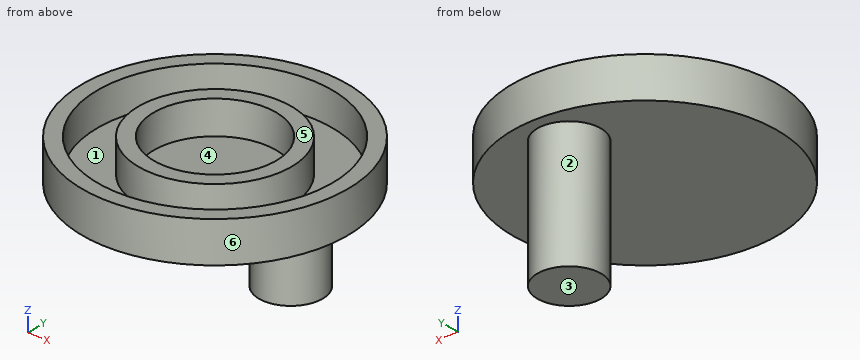
```python
from build123d import *

# Parameters (mm, degrees)
SKETCH1_R           = 12.5
BOSS_EXTRUDE1_DEPTH = 50
SKETCH2_R           = 52.025
SKETCH2_R_2         = 46.025
SKETCH2_R_3         = 29.975
SKETCH2_R_4         = 23.975
BOSS_EXTRUDE2_DEPTH = 16
SKETCH4_R           = 52.025
BOSS_EXTRUDE3_DEPTH = 3


with BuildPart() as part:
    # Sketch1 → Boss-Extrude1 (new body)
    with BuildSketch(Plane.XY):
        Circle(SKETCH1_R)
    extrude(amount=-BOSS_EXTRUDE1_DEPTH)

    # Sketch2 → Boss-Extrude2 (add)
    with BuildSketch(Plane.XY):
        with Locations((0, -35)):
            Circle(SKETCH2_R)
        with Locations((0, -35)):
            Circle(SKETCH2_R_2, mode=Mode.SUBTRACT)
        with Locations((0, -35)):
            Circle(SKETCH2_R_3)
        with Locations((0, -35)):
            Circle(SKETCH2_R_4, mode=Mode.SUBTRACT)
    extrude(amount=BOSS_EXTRUDE2_DEPTH)

    # Sketch4 → Boss-Extrude3 (add)
    with BuildSketch(Plane.XY):
        with Locations((0, -35)):
            Circle(SKETCH4_R)
    extrude(amount=BOSS_EXTRUDE3_DEPTH)


solid = part.part
```
Geometry check sheet. Reference: the model listing, model coordinates, mm. Face numbers are marked on the shaded views. A direction names the side the tool comes from. Round coordinates to 2 decimals unless told otherwise and drop trailing zeros. Order: outer loops, then holes, each group sorted by start corner. A loop starts at its lowest first (then second) coordinate and runs counter-clockwise, first axis right, second up. Notation, with made-up numbers: M 60.5,-15.75 L 119.5,-15.75 A9 ccw 119.5,-8.75 Z; hole C 55,58 d2. An arc over 180 degrees is marked long. Write item = value, one per line.
Q1. Release check for a two-part mould opening along X. For the marked faces 4, 5 and 6 record: released by +X, released by -X, zero draft, split by the parting line, or undercut.
Answer block:
face_4 = undercut
face_5 = zero draft
face_6 = split by the parting line
Q2. Section check C-C (z = 1.5). Enter the section's corners in (x, y) (3 decimals), plus the area to 3 significant figures.
Answer block:
outline = C 0,-35 d104.05
area = 8,500 mm^2
Q3. Scan lines: line 1 (Y direction, x = 0, z = 10) (3 decimals); line 2 (X direction, y = -51, z = 12.5); line 3 (X direction, y = -9, z = 10.5). Record each from-to range of solid material in increasing order.
Answer block:
line_1 = -87.025 to -81.025, -64.975 to -58.975, -11.025 to -5.025, 11.025 to 17.025
line_2 = -49.5 to -43.15, -25.35 to -17.85, 17.85 to 25.35, 43.15 to 49.5
line_3 = -45.06 to -37.98, -14.92 to 14.92, 37.98 to 45.06
Q4. Section check D-D (y = 2). Enter the section's corners in (x, z), plus the area to 3 significant figures.
Answer block:
outline = M -36.57,0 L -12.34,0 L -12.34,-50 L 12.34,-50 L 12.34,0 L 36.57,0 L 36.57,16 L 27.37,16 L 27.37,3 L -27.37,3 L -27.37,16 L -36.57,16 Z
area = 1,690 mm^2
Q5. Depth check by flat-ended pin: pin 1 Ø8 at (x, y) = (-27.5, -35.5) entering from -Z; pin 2 Ø3 at (x, y) = (-9, -44) entering from +Z; pin 3 Ø10 at (y, z) = (-11.5, -2.5) entering from -X; pin 4 Ø12 at (y, z) = (-19, -30.5) entering from -X. Enter the tip coordinate at first touch or a pass-through.
Answer block:
pin_1 = 0
pin_2 = 3
pin_3 = -48.36
pin_4 = through
Q6. Section check A-A (y = -35). Enter the section's corners in (x, z) (3 decimals), plus the area to 3 significant figures.
Answer block:
outline = M -52.025,0 L 52.025,0 L 52.025,16 L 46.025,16 L 46.025,3 L 29.975,3 L 29.975,16 L 23.975,16 L 23.975,3 L -23.975,3 L -23.975,16 L -29.975,16 L -29.975,3 L -46.025,3 L -46.025,16 L -52.025,16 Z
area = 624 mm^2
Q7. Set-up check for the marked faces 1, 2 and 3: record each of +Z, -Z, +X, -X, +Y, -Y from which the full face is reachable in a straight line by a thin tool's end or side.
Answer block:
face_1 = +Z
face_2 = -Z
face_3 = -Z, +X, -X, +Y, -Y
Q8. Section check B-B (x = 0). Enter the section's corners in (y, z) (3 decimals), plus the area to 3 significant figures.
Answer block:
outline = M -87.025,0 L -12.5,0 L -12.5,-50 L 12.5,-50 L 12.5,0 L 17.025,0 L 17.025,16 L 11.025,16 L 11.025,3 L -5.025,3 L -5.025,16 L -11.025,16 L -11.025,3 L -58.975,3 L -58.975,16 L -64.975,16 L -64.975,3 L -81.025,3 L -81.025,16 L -87.025,16 Z
area = 1,870 mm^2
